Design review of the part built by this model. Coordinates are the model's own, in mm. A direction names the side the tool comes from. Give positions to 0.01 mm unless a question says otherwise; leave off trailing zeros. Write each loop counter-clockwise with the first axis right and the second up, starting at its lowest first coordinate (ties: lowest second). Pieces come first, ordered by that corner, then holes. Notation, with made-up numbers: (-36, -30) -> (19, -30) arc R3 ccw to (19, -26) -> close; hole circle Ø1 at (-30, 84). An arc over 180 degrees is marked (long way). Answer as a JSON object with one key per item and string values.
```python
from build123d import *

# Parameters (mm, degrees)
SKETCH1_W           = 38.1
SKETCH1_H           = 6.096
BOSS_EXTRUDE1_DEPTH = 22.86
SKETCH4_W           = 25.4
SKETCH4_H           = 6.096
CUT_EXTRUDE1_DEPTH  = 15.875
FILLET1_R           = 1.27
SKETCH5_W           = 38.1
SKETCH5_H           = 19.685
BOSS_EXTRUDE2_DEPTH = 5.08
BOSS_EXTRUDE3_DEPTH = 6.096
BOSS_EXTRUDE4_DEPTH = 6.096
FILLET2_R           = 1.27
SKETCH9_W           = 38.1
SKETCH9_H           = 5.08
BOSS_EXTRUDE5_DEPTH = 22.86
SKETCH10_W          = 8.509
SKETCH10_H          = 17.78
BOSS_EXTRUDE6_DEPTH = 5.08
SKETCH11_W          = 8.509
SKETCH11_H          = 17.78
BOSS_EXTRUDE7_DEPTH = 5.08
SKETCH12_W          = 19.05
SKETCH12_H          = 7.62
CUT_EXTRUDE2_DEPTH  = 5.08
FILLET3_R           = 2.54
FILLET5_R           = 2.54
FILLET6_R           = 1.27
SKETCH13_W          = 13.940844751
SKETCH13_H          = 3.429
BOSS_EXTRUDE8_DEPTH = 1.524
CUT_EXTRUDE5_REACH  = 52.09
SKETCH22_W          = 1.778
SKETCH22_H          = 5.08
FILLET7_R           = 0.635


with BuildPart() as part:
    # Sketch1 → Boss-Extrude1 (new body)
    with BuildSketch(Plane(origin=(0, 0, 0), x_dir=(1, 0, 0), z_dir=(0, 1, 0))):
        Rectangle(SKETCH1_W, SKETCH1_H)
    extrude(amount=BOSS_EXTRUDE1_DEPTH)

    # Sketch4 → Cut-Extrude1 (cut)
    with BuildSketch(Plane.XZ):
        Rectangle(SKETCH4_W, SKETCH4_H)
    extrude(amount=-CUT_EXTRUDE1_DEPTH, mode=Mode.SUBTRACT)

    # Fillet1
    fillet1_edges = [part.edges().sort_by_distance(p)[0] for p in [
        (0, 15.875, -3.048),
    ]]
    fillet(fillet1_edges, radius=FILLET1_R)

    # Sketch5 → Boss-Extrude2 (add)
    with BuildSketch(Plane(origin=(0, 22.86, 0), x_dir=(1, 0, 0), z_dir=(0, 1, 0))):
        with Locations((0, -6.7945)):
            Rectangle(SKETCH5_W, SKETCH5_H)
    extrude(amount=BOSS_EXTRUDE2_DEPTH)

    # Sketch6 → Boss-Extrude3 (add)
    with BuildSketch(Plane.XY.offset(3.048)):
        Polygon((-12.7, 0), (-10.668, 0), (-12.7, 6.858), align=None)
    extrude(amount=-BOSS_EXTRUDE3_DEPTH)

    # Sketch7 → Boss-Extrude4 (add)
    with BuildSketch(Plane.XY.offset(3.048)):
        Polygon((12.7, 0), (10.668, 0), (12.7, 6.858), align=None)
    extrude(amount=-BOSS_EXTRUDE4_DEPTH)

    # Fillet2
    fillet2_edges = [part.edges().sort_by_distance(p)[0] for p in [
        (-10.668, 0, 0),
        (10.668, 0, 0),
    ]]
    fillet(fillet2_edges, radius=FILLET2_R)

    # Sketch9 → Boss-Extrude5 (add)
    with BuildSketch(Plane.XZ.offset(-22.86)):
        with Locations((0, 14.097)):
            Rectangle(SKETCH9_W, SKETCH9_H)
    extrude(amount=BOSS_EXTRUDE5_DEPTH)

    # Sketch10 → Boss-Extrude6 (add)
    with BuildSketch(Plane(origin=(19.05, 0, 0), x_dir=(0, 0, -1), z_dir=(1, 0, 0))):
        with Locations((-7.3025, 8.89)):
            Rectangle(SKETCH10_W, SKETCH10_H)
    extrude(amount=-BOSS_EXTRUDE6_DEPTH)

    # Sketch11 → Boss-Extrude7 (add)
    with BuildSketch(Plane.ZY.offset(19.05)):
        with Locations((7.3025, 8.89)):
            Rectangle(SKETCH11_W, SKETCH11_H)
    extrude(amount=-BOSS_EXTRUDE7_DEPTH)

    # Sketch12 → Cut-Extrude2 (cut)
    with BuildSketch(Plane.XY.offset(16.637)):
        with Locations((0, 19.05)):
            Rectangle(SKETCH12_W, SKETCH12_H)
    extrude(amount=-CUT_EXTRUDE2_DEPTH, mode=Mode.SUBTRACT)

    # Fillet3
    fillet3_edges = [part.edges().sort_by_distance(p)[0] for p in [
        (9.525, 22.86, 14.097),
        (9.525, 15.24, 14.097),
        (-9.525, 15.24, 14.097),
        (-9.525, 22.86, 14.097),
    ]]
    fillet(fillet3_edges, radius=FILLET3_R)

    # Fillet5
    fillet5_edges = [part.edges().sort_by_distance(p)[0] for p in [
        (13.0175, 22.86, 11.557),
        (16.51, 17.78, 11.557),
        (16.51, 17.78, 3.048),
        (0, 22.86, 3.048),
        (-13.0175, 22.86, 11.557),
        (-16.51, 17.78, 11.557),
        (-16.51, 17.78, 3.048),
    ]]
    fillet(fillet5_edges, radius=FILLET5_R - 0.0001)  # a hair under: the kernel refuses the full size

    # Fillet6
    fillet6_edges = [part.edges().sort_by_distance(p)[0] for p in [
        (19.05, 13.97, 16.637),
        (-19.05, 13.97, 16.637),
        (19.05, 27.94, 6.7945),
        (0, 27.94, -3.048),
        (-19.05, 27.94, 6.7945),
        (0, 27.94, 16.637),
        (-19.05, 0, 6.7945),
        (19.05, 0, 6.7945),
        (-19.05, 13.97, -3.048),
        (19.05, 13.97, -3.048),
        (0, 0, 16.637),
    ]]
    fillet(fillet6_edges, radius=FILLET6_R)

    # Sketch13 → Boss-Extrude8 (add)
    with BuildSketch(Plane.XZ.offset(-22.86)):
        with Locations((-0.014577624, 7.3025)):
            Rectangle(SKETCH13_W, SKETCH13_H)
    extrude(amount=BOSS_EXTRUDE8_DEPTH)

    # Cut-Extrude5: up to this face of the body (flat: up to its plane)
    cut_extrude5_end = Plane(part.part.faces().sort_by_distance((-19.05, 13.368385641, 6.746370851))[0])
    # Sketch22 → Cut-Extrude5 (cut, up to the picked face)
    with BuildSketch(Plane(origin=(19.05, 0, 0), x_dir=(0, 0, -1), z_dir=(1, 0, 0)), mode=Mode.PRIVATE) as cut_extrude5_sk1:
        with Locations((-9.982963742, 5.043439789)):
            Rectangle(SKETCH22_W, SKETCH22_H)
    cut_extrude5_tool1 = split(extrude(cut_extrude5_sk1.sketch, amount=-CUT_EXTRUDE5_REACH, mode=Mode.PRIVATE), bisect_by=cut_extrude5_end, keep=Keep.BOTH, mode=Mode.PRIVATE)
    add(cut_extrude5_tool1.solids().sort_by(Axis((19.05, 5.04344, 9.982964), (-1, 0, 0)))[0], mode=Mode.SUBTRACT)

    # Fillet7
    fillet7_edges = [part.edges().sort_by_distance(p)[0] for p in [
        (16.51, 2.503439789, 10.871963742),
        (16.51, 7.583439789, 10.871963742),
        (16.51, 7.583439789, 9.093963742),
        (16.51, 2.503439789, 9.093963742),
        (-16.51, 2.503439789, 10.871963742),
        (-16.51, 7.583439789, 10.871963742),
        (-16.51, 7.583439789, 9.093963742),
        (-16.51, 2.503439789, 9.093963742),
    ]]
    fillet(fillet7_edges, radius=FILLET7_R)


solid = part.part
```
(1) We need section C-C, the plane z = 13.25. State the section outline as (x, y) points (3 decimals), then the cut area to 3 significant figures.
Here are the results:
{"outline": "(-19.05, 1.27) arc R1.27 ccw to (-17.78, 0) -> (17.78, 0) arc R1.27 ccw to (19.05, 1.27) -> (19.05, 26.67) arc R1.27 ccw to (17.78, 27.94) -> (-17.78, 27.94) arc R1.27 ccw to (-19.05, 26.67) -> close; hole (-9.525, 17.78) arc R2.54 ccw to (-6.985, 15.24) -> (6.985, 15.24) arc R2.54 ccw to (9.525, 17.78) -> (9.525, 20.32) arc R2.54 ccw to (6.985, 22.86) -> (-6.985, 22.86) arc R2.54 ccw to (-9.525, 20.32) -> close", "area": "924 mm²"}
(2) The part is to be moulded in two halves that separate along Z. For faces 6 (the cylindrical face through (-8.761, 22.136, 13.62)), 7 (the flat face through (-16, 5, 9.094)), 8 (the cylindrical face through (16.474, 18.544, 3.772)), 9 (the cylindrical face through (0.249, 27.558, 16.275)), say which applies: +Z half, -Z half, draft (parallel to the pull), parting line (faces both ways), or undercut.
Here are the results:
{"face 6": "draft", "face 7": "undercut", "face 8": "undercut", "face 9": "+Z half"}
(3) For faces 1 (the flat face through (-6.985, 22, 7)), 2 (the flat face through (-16, 5, 10.872)), 3 (the flat face through (0, 22.86, 10)), 4 (the cylindrical face through (8.761, 15.964, 14.061)), 5 (the flat face through (0, 21.336, 7)), list the 3-axis set-ups (+Z, -Z, +X, -X, +Y, -Y) from which the entire face can be reached by the end or side of a thin tool; tool diameter is ignored.
Here are the results:
{"face 1": "+Z, -X, -Y", "face 2": "+X, -X", "face 3": "none", "face 4": "+Z", "face 5": "+Z, +X, -X, -Y"}
(4) For line 1 along X through (y, z) = (17.25, 10.25); line 2 along Y through (x, z) = (-1.5, 13.5); line 3 along X through (y, z) = (7, -1), list the stretches that pass through material, from the lowest coordinate up.
Here are the results:
{"line 1": "x = -19.05 to -13.97, 13.97 to 19.05", "line 2": "y = 0 to 15.24, 22.86 to 27.94", "line 3": "x = -19.05 to -12.7, 12.7 to 19.05"}
(5) We need section B-B, the plane x = 16. Give the number of separate pieces and of enclosed holes in the cut face, then the cut area to 3 significant figures.
Here are the results:
{"separate pieces": "1", "enclosed holes": "2", "area": "503 mm²"}
(6) We need section A-A, the plane z = 7. State the section outline as (x, y) points (3 decimals).
Here are the results:
{"outline": "(-19.05, 1.27) arc R1.27 ccw to (-17.78, 0) -> (-13.97, 0) -> (-13.97, 17.78) -> (-19.05, 17.78) -> close; (-19.05, 22.86) -> (-6.985, 22.86) -> (-6.985, 21.336) -> (6.956, 21.336) -> (6.956, 22.86) -> (19.05, 22.86) -> (19.05, 26.67) arc R1.27 ccw to (17.78, 27.94) -> (-17.78, 27.94) arc R1.27 ccw to (-19.05, 26.67) -> close; (13.97, 0) -> (17.78, 0) arc R1.27 ccw to (19.05, 1.27) -> (19.05, 17.78) -> (13.97, 17.78) -> close"}
(7) Clearance check with flat-ended pins moving along their axes: pin 1 (1 mm diameter, centred on x = 2.5, z = 6.5, fed in from -Y); pin 2 (0.5 mm diameter, centred on y = 22.5, z = 7, fed in from +X). State where each tip first meets the part, or that it passes through.
Here are the results:
{"pin 1": "stops at y = 21.34", "pin 2": "stops at x = 6.96"}
(8) We need section D-D, the plane y = 5.25. State the section outline as (x, z) points, then the cut area to 3 significant figures.
Here are the results:
{"outline": "(-19.05, -1.78) arc R1.27 ccw to (-17.78, -3.05) -> (-12.22, -3.05) -> (-12.22, 3.05) -> (-13.97, 3.05) -> (-13.97, 9.09) -> (-19.05, 9.09) -> close; (-19.05, 10.87) -> (-13.97, 10.87) -> (-13.97, 11.56) -> (13.97, 11.56) -> (13.97, 10.87) -> (19.05, 10.87) -> (19.05, 15.37) arc R1.27 ccw to (17.78, 16.64) -> (-17.78, 16.64) arc R1.27 ccw to (-19.05, 15.37) -> close; (12.22, -3.05) -> (17.78, -3.05) arc R1.27 ccw to (19.05, -1.78) -> (19.05, 9.09) -> (13.97, 9.09) -> (13.97, 3.05) -> (12.22, 3.05) -> close", "area": "344 mm²"}
